For this review, use the dimensioned drawing (mm, ordinates from the lowest corner) and the shaded views. A direction names the side the tool comes from. Coordinates: 2 decimals unless noted, no trailing zeros. Order: outer loops, then holes, each group sorted by start corner. A loop starts at its lowest first (then second) coordinate and runs counter-clockwise, first axis right, second up. Notation, with made-up numbers: (-18, 7) -> (-9, 7) arc R25 cw to (-9, 33) -> close; hole circle Ø8 at (-7, 71.25). An arc over 180 degrees is marked (long way). Use one line per item in the form item = value. Start each with the question number.
(1) Take a section at B-B (z = 10.5). State the section outline as (x, y) points.
(2) Take a section at A-A (y = 2.75). State the section outline as (x, z) points.
(3) Mouldability with a two-part tool opening along Y and no side actions: class the marked faces 3, 4 and 5 as +Y half, -Y half, draft (parallel to the pull), parting line (faces both ways), or undercut.
(4) For the marked faces 1 and 2, list the 3-axis set-ups (+Z, -Z, +X, -X, +Y, -Y) from which the entire face can be reached by the end or side of a thin tool; tool diameter is ignored.
(5) Take a section at D-D (y = 5.1). State the section outline as (x, z) points.
(6) Wall thickness on line 1 along Z through (x, y) = (1.95, 3.15); line 2 along Z through (x, y) = (1.45, 3.7); line 3 along Y through (x, z) = (2.75, 11.5): over which ranges is each line inside the solid? List them lowest first.
(7) Take a section at C-C (x = 2.4). State the section outline as (y, z) points.
(8) Insertion check: pin 1 Ø1.5 at (x, y) = (3, 4) entering from -Z; pin 2 Ø1.5 at (x, z) = (2, 9.5) entering from -Y; pin 3 Ø2 at (y, z) = (2.5, 9.5) entering from +X; pin 4 Ø1.2 at (x, y) = (3, 3) entering from +Z. Each pin has a flat end and moves straight along its axis. Give the tip position at first contact, or say it passes through.
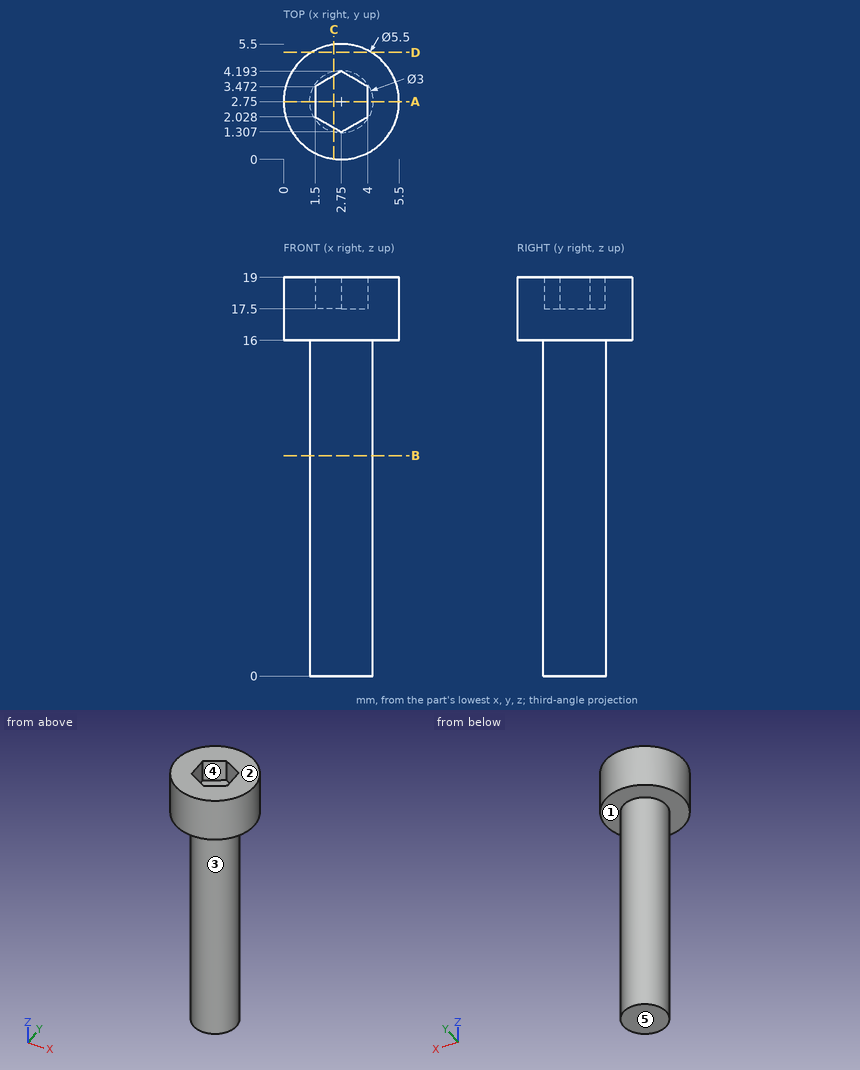
Findings:
q1.outline = circle Ø3 at (2.75, 2.75)
q2.outline = (0, 16) -> (1.25, 16) -> (1.25, 0) -> (4.25, 0) -> (4.25, 16) -> (5.5, 16) -> (5.5, 19) -> (4, 19) -> (4, 17.5) -> (1.5, 17.5) -> (1.5, 19) -> (0, 19) -> close
q3.face_3 = parting line
q3.face_4 = undercut
q3.face_5 = draft
q4.face_1 = -Z
q4.face_2 = +Z, +X, -X, +Y, -Y
q5.outline = (1.32, 16) -> (4.18, 16) -> (4.18, 19) -> (1.32, 19) -> close
q6.line_1 = 0 to 17.5
q6.line_2 = 16 to 19
q6.line_3 = 1.25 to 4.25
q7.outline = (0.02, 16) -> (1.29, 16) -> (1.29, 0) -> (4.21, 0) -> (4.21, 16) -> (5.48, 16) -> (5.48, 19) -> (3.99, 19) -> (3.99, 17.5) -> (1.51, 17.5) -> (1.51, 19) -> (0.02, 19) -> close
q8.pin_1 = 0
q8.pin_2 = 1.25
q8.pin_3 = 4.25
q8.pin_4 = 17.5
